Build history of the part. All positions in model axes, mm. A direction names the side the tool comes from. Coordinates: 2 decimals unless noted, no trailing zeros. Write each loop counter-clockwise with the first axis right and the second up, starting at its lowest first coordinate (ties: lowest second). Pieces come first, ordered by that corner, then holes. Notation, with made-up numbers: (27, -28) -> (46, -28) arc R18 ccw to (46, 2) -> close; hole circle Ø11 at (52, -15). An arc over 180 degrees is marked (long way). Write each question's results on one line, items separated by ' | '. Start each with the question number.
Q1. Tool access for faces 4 (the face through (-33.24, 1.61, -36.83)), 5 (the face through (-16, 3.175, 16)): list every direction of +Z, -Z, +X, -X, +Y, -Y with a clear straight run to the whole face (end or side of a thin tool).
Q2. Saw through at B-B on x = -7. Give the cut face in (y, z) (3 decimals).
Q3. Saw through at C-C on z = 16. Give the cut face in (x, y) (3 decimals), and give its area (3 significant figures).
Q4. Saw through at D-D on z = 39.5. Give the cut face in (x, y) (3 decimals), and give its area (3 significant figures).
Q5. Two-plate mould, pull along X, no slides. Class faces 1 (the face through (-16, 0, 16)), 2 (the face through (23.27, 1.57, 73.88)), 3 (the face through (-26.63, 1.61, -27)): released by +X, released by -X, zero draft, split by the parting line, or undercut.
Q6. Drill centre lines: line 1 (X direction, y = 0.95, z = 0); line 2 (X direction, y = 2.1, z = -33.02); line 3 (Z direction, x = -18.5, y = 1). Where is each one in solid material? Low to high.
Q7. Saw through at A-A on y = 2.5. Give the cut face in (x, z), and give its area (3 significant figures).
from build123d import *

# Parameters (mm, degrees)
SKETCH1_R           = 77.4600051
BOSS_EXTRUDE1_DEPTH = 3.175
SKETCH24_R          = 22.1615
SKETCH24_R_2        = 2.0193
CUT_EXTRUDE14_DEPTH = 110.590991442


with BuildPart() as part:
    # Sketch1 → Boss-Extrude1 (new body)
    with BuildSketch(Plane(origin=(0, 0, 0), x_dir=(1, 0, 0), z_dir=(0, 1, 0))):
        with Locations(Location((0, 0, 0), (0, 0, 270))):
            Circle(SKETCH1_R)
    extrude(amount=BOSS_EXTRUDE1_DEPTH)

    # Sketch24 → Cut-Extrude14 (cut, through all)
    with BuildSketch(Plane(origin=(0, 3.175, 0), x_dir=(1, 0, 0), z_dir=(0, 1, 0))):
        with Locations(Location((0, 0, 0), (0, 0, 270))):
            Circle(SKETCH24_R)
        with Locations(Location((-25.4, 25.4, 0), (0, 0, 270))):
            Circle(SKETCH24_R_2)
        with Locations(Location((0, 33.02, 0), (0, 0, 270))):
            Circle(SKETCH24_R_2)
        with Locations(Location((33.02, 0, 0), (0, 0, 270))):
            Circle(SKETCH24_R_2)
        with Locations(Location((0, -33.02, 0), (0, 0, 270))):
            Circle(SKETCH24_R_2)
        with Locations(Location((-33.02, 0, 0), (0, 0, 270))):
            Circle(SKETCH24_R_2)
        with BuildLine():
            Line((-32.276051224, 28.683948776), (-41.256307345, 37.664204897))
            ThreePointArc((-41.256307345, 37.664204897), (-41.256307345, 41.256307345), (-37.664204897, 41.256307345))
            Line((-37.664204897, 41.256307345), (-28.683948776, 32.276051224))
            ThreePointArc((-28.683948776, 32.276051224), (-28.683948776, 28.683948776), (-32.276051224, 28.683948776))
        make_face()
    extrude(amount=-CUT_EXTRUDE14_DEPTH, mode=Mode.SUBTRACT)


solid = part.part
Returned:
1) face 4: +Y, -Y | face 5: +Z, -Z, +X, -X, +Y
2) outline: (0, -77.143) -> (3.175, -77.143) -> (3.175, -21.027) -> (0, -21.027) -> close; (0, 21.027) -> (3.175, 21.027) -> (3.175, 77.143) -> (0, 77.143) -> close
3) outline: (-75.79, 0) -> (-15.334, 0) -> (-15.334, 3.175) -> (-75.79, 3.175) -> close; (15.334, 0) -> (75.79, 0) -> (75.79, 3.175) -> (15.334, 3.175) -> close | area: 384 mm2
4) outline: (-66.632, 0) -> (66.632, 0) -> (66.632, 3.175) -> (-66.632, 3.175) -> close | area: 423 mm2
5) face 1: zero draft | face 2: split by the parting line | face 3: undercut
6) line 1: x = -77.46 to -35.04, -31 to -22.16, 22.16 to 31, 35.04 to 77.46 | line 2: x = -70.07 to -36.61, -29.43 to -2.02, 2.02 to 70.07 | line 3: z = -75.22 to -12.2, 12.2 to 75.22
7) outline: circle Ø154.92 at (0, 0); hole (-41.26, -37.66) arc R2.54 ccw to (-37.66, -41.26) -> (-28.68, -32.28) arc R2.54 ccw to (-32.28, -28.68) -> close; hole circle Ø4.04 at (-33.02, 0); hole circle Ø4.04 at (-25.4, -25.4); hole circle Ø44.32 at (0, 0); hole circle Ø4.04 at (0, -33.02); hole circle Ø4.04 at (0, 33.02); hole circle Ø4.04 at (33.02, 0) | area: 17,200 mm2
